Source: CAD feature listing. Evaluate the final solid. Frame: model axes, mm. Face numbers are marked on the shaded views. A direction names the side the tool comes from. Give positions to 0.01 mm unless a question says otherwise; leave off trailing zeros. Order: outer loops, then holes, each group sorted by start corner. A loop starts at its lowest first (then second) coordinate and runs counter-clockwise, first axis right, second up. Notation, with made-up numbers: (3, 79.5) - (32, 79.5) arc R5 cw to (32, 87.5) - close; hole circle Ø5 at (71.5, 71.25). An arc over 180 degrees is marked (long way). Use CSV: the item, a comma, the result in double quotes.
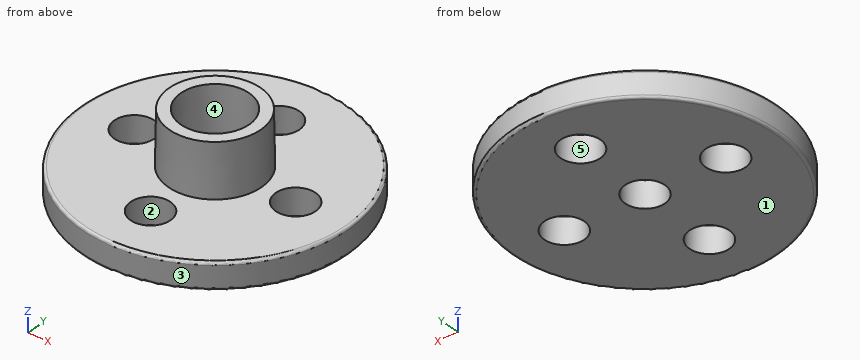
```python
from build123d import *

# Parameters (mm, degrees)
IZIM1_R                     = 10
IZIM1_R_2                   = 1.5
Y_KSEKLIK_EKSTR_ZYON1_DEPTH = 2
RADYUS1_R                   = 0.2
IZIM2_R                     = 3.5
IZIM2_R_2                   = 2.5
Y_KSEKLIK_EKSTR_ZYON2_DEPTH = 4
Y_KSEKLIK_EKSTR_ZYON2_TAPER = 1
IZIM3_R                     = 1.5
KES_EKSTR_ZYON1_DEPTH       = 4


with BuildPart() as part:
    # Çizim1 → Yükseklik-Ekstrüzyon1 (new body)
    with BuildSketch(Plane.XY):
        Circle(IZIM1_R)
        with Locations((0, 6)):
            Circle(IZIM1_R_2, mode=Mode.SUBTRACT)
        with Locations((6, 0)):
            Circle(IZIM1_R_2, mode=Mode.SUBTRACT)
        with Locations((0, -6)):
            Circle(IZIM1_R_2, mode=Mode.SUBTRACT)
        with Locations((-6, 0)):
            Circle(IZIM1_R_2, mode=Mode.SUBTRACT)
    extrude(amount=Y_KSEKLIK_EKSTR_ZYON1_DEPTH)

    # Radyus1
    radyus1_edges = [part.edges().sort_by_distance(p)[0] for p in [
        (-10, 0, 0),
        (-10, 0, 2),
    ]]
    fillet(radyus1_edges, radius=RADYUS1_R)

    # Çizim2 → Yükseklik-Ekstrüzyon2 (add)
    with BuildSketch(Plane.XY.offset(2)):
        Circle(IZIM2_R)
        Circle(IZIM2_R_2, mode=Mode.SUBTRACT)
    extrude(amount=Y_KSEKLIK_EKSTR_ZYON2_DEPTH, taper=Y_KSEKLIK_EKSTR_ZYON2_TAPER)

    # Çizim3 → Kes-Ekstrüzyon1 (cut)
    with BuildSketch(Plane(origin=(0, 0, 0), x_dir=(-1, 0, 0), z_dir=(0, 0, -1))):
        Circle(IZIM3_R)
    extrude(amount=-KES_EKSTR_ZYON1_DEPTH, mode=Mode.SUBTRACT)


solid = part.part
```
Item 1: Material intervals for line 1 (Y direction, x = 0, z = 1.45); line 2 (Z direction, x = -2.25, y = 7.5); line 3 (Y direction, x = 6, z = 1.15), sorted ascending. Write a range as from..to.
Filled in:
line 1,"y = -10..-7.5, -4.5..-1.5, 1.5..4.5, 7.5..10"
line 2,"z = 0..2"
line 3,"y = -8..-1.5, 1.5..8"
Item 2: Mould query, pull axis X, two halves, no side actions, for the marked faces 1, 2 and 3. Classes: released by +X, released by -X, zero draft, split by the parting line, or undercut.
Filled in:
face 1,"zero draft"
face 2,"undercut"
face 3,"split by the parting line"
Item 3: First-contact query: pin 1 (3 mm diameter, centred on y = -1.5, z = 3, fed in from +X); pin 2 (3.5 mm diameter, centred on x = 6, y = 0, fed in from +Z). Flat tips, straight axial feed; report the tip coordinate or a pass-through.
Filled in:
pin 1,"stops at x = 9.98"
pin 2,"stops at z = 2"
Item 4: Section D-D on z = 3. Return the cut outline in (x, y), then the cut area to 3 significant figures.
Filled in:
outline,"circle Ø6.97 at (0, 0); hole circle Ø5.03 at (0, 0)"
area,"18.2 mm2"
Item 5: Set-up query: the marked faces 4 and 5. Return all of +Z, -Z, +X, -X, +Y, -Y with unobstructed straight access to the full face (end or side cutting, diameter ignored); none if empty.
Filled in:
face 4,"+Z"
face 5,"+Z, -Z"
Item 6: Section B-B on y = 0. Count the separate pieces of the cut face and the enclosed holes in it, then the cut area to 3 significant figures.
Filled in:
separate pieces,"4"
enclosed holes,"0"
area,"29.4 mm2"
Item 7: Section A-A on z = 0.5. Return the cut outline in (x, y), then the cut area to 3 significant figures.
Filled in:
outline,"circle Ø20 at (0, 0); hole circle Ø3 at (-6, 0); hole circle Ø3 at (0, -6); hole circle Ø3 at (0, 0); hole circle Ø3 at (0, 6); hole circle Ø3 at (6, 0)"
area,"279 mm2"
